Answer from the drawing. Dimensions are ordinates in mm from the lowest x, y and z of the part. A direction names the side the tool comes from. Round coordinates to 2 decimals unless told otherwise and drop trailing zeros. Loops run counter-clockwise (first coordinate to the right, second up) from the corner with the lowest first, then second, coordinate; pieces in that order, holes last. Notation, with made-up numbers: M 77.5,13.25 L 129.5,13.25 A16 cw 129.5,31.25 Z; hole C 24,52 d9. An arc over 180 degrees is marked long. Write each question's results on one line, items separated by ' | '.
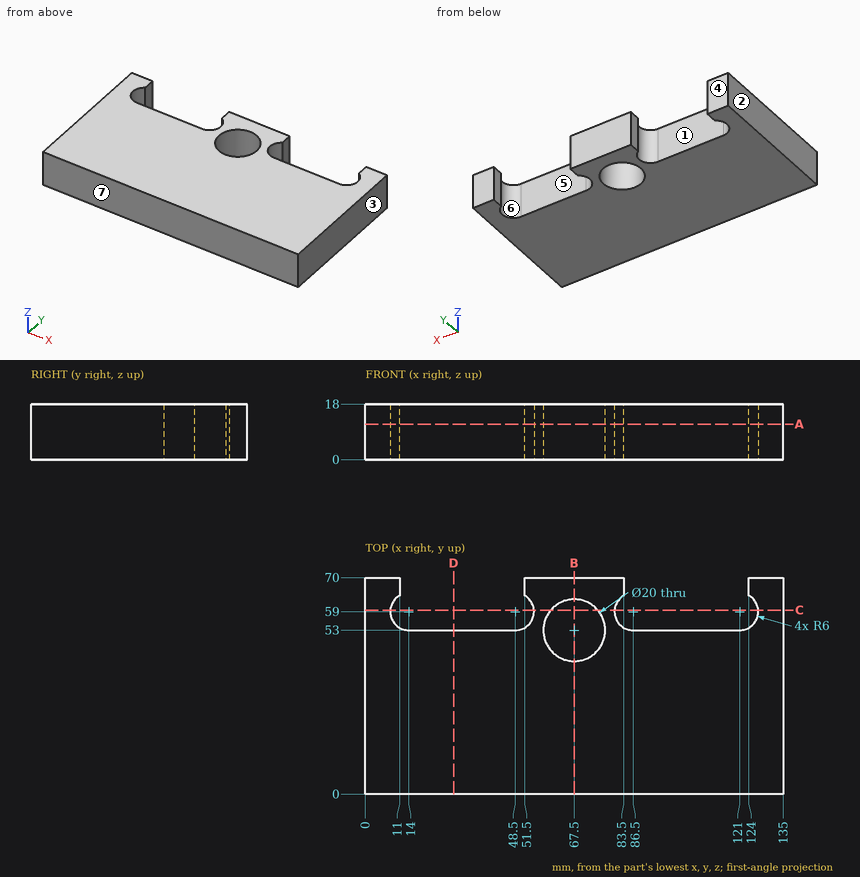
1. Determine the mould class of the marked faces 1, 2, 3 and 4 for opening direction X: released by +X, released by -X, zero draft, split by the parting line, or undercut.
Completed:
face 1: undercut | face 2: released by -X | face 3: released by +X | face 4: zero draft
2. Find the intervals of material crossed by L1, parallel to Y at x = 67.5, z = 5.75; L2, parallel to Y at x = 104, z = 17; L3, parallel to Y at x = 64, z = 3.5, in increasing order.
Completed:
L1: y = 0 to 43, 63 to 70 | L2: y = 0 to 53 | L3: y = 0 to 43.63, 62.37 to 70
3. Which of the six approach directions +Z, -Z, +X, -X, +Y, -Y give full straight-line access (tool end or side, diameter ignored) to the marked faces 5, 6 and 7?
Completed:
face 5: +Z, -Z, +Y | face 6: +Z, -Z | face 7: +Z, -Z, +X, -X, -Y
4. Given P1, Ø18, axis at x = 67.5, y = 53, coming from the -Z side, flat-ended and moving along its own axis, determine where the tip first touches the part or whether it passes through.
Completed:
P1: passes through
5. Find section A-A, the plane z = 11.5. Give the vertices of the cut face in (x, y), then the cut area to 3 significant figures.
Completed:
outline: M 0,0 L 135,0 L 135,70 L 124,70 L 124,64.2 A6 cw 121,53 L 86.5,53 A6 cw 83.5,64.2 L 83.5,70 L 51.5,70 L 51.5,64.2 A6 cw 48.5,53 L 14,53 A6 cw 11,64.2 L 11,70 L 0,70 Z; hole C 67.5,53 d20 | area: 7,670 mm2
6. Find section C-C, the plane y = 59.5. Give the vertices of the cut face in (x, z).
Completed:
outline: M 0,0 L 8.02,0 L 8.02,18 L 0,18 Z; M 54.48,0 L 59.9,0 L 59.9,18 L 54.48,18 Z; M 75.1,0 L 80.52,0 L 80.52,18 L 75.1,18 Z; M 126.98,0 L 135,0 L 135,18 L 126.98,18 Z
7. Find section D-D, the plane x = 28.5. Give the vertices of the cut face in (y, z).
Completed:
outline: M 0,0 L 53,0 L 53,18 L 0,18 Z
8. Find section B-B, the plane x = 67.5. Give the vertices of the cut face in (y, z).
Completed:
outline: M 0,0 L 43,0 L 43,18 L 0,18 Z; M 63,0 L 70,0 L 70,18 L 63,18 Z
